CAD build for the part. Positions are in the model's coordinates, mm. Give positions to 0.01 mm unless a question says otherwise; leave off trailing zeros. Loops run counter-clockwise (first coordinate to the right, second up) from the corner with the lowest first, then second, coordinate; pieces in that order, holes last. Notation, with made-up numbers: (44, 43) -> (86, 43) arc R25 cw to (86, 76) -> close; hole circle Ø2 at (50, 19). An arc over 180 degrees is marked (long way). Use one line per item in the form item = value.
```python
from build123d import *

# Parameters (mm, degrees)
SKETCH1_W           = 245
SKETCH1_H           = 65
BOSS_EXTRUDE1_DEPTH = 3
CUT_EXTRUDE1_DEPTH  = 10
SKETCH3_W           = 3
SKETCH3_H           = 12.5
CUT_EXTRUDE2_DEPTH  = 10
SKETCH5_W           = 12
SKETCH5_H           = 3
SKETCH5_W_2         = 13.071416553
BOSS_EXTRUDE2_DEPTH = 3


with BuildPart() as part:
    # Sketch1 → Boss-Extrude1 (new body)
    with BuildSketch(Plane(origin=(0, 0, 0), x_dir=(1, 0, 0), z_dir=(0, 1, 0))):
        Rectangle(SKETCH1_W, SKETCH1_H)
    extrude(amount=BOSS_EXTRUDE1_DEPTH)

    # Sketch2 → Cut-Extrude1 (cut)
    with BuildSketch(Plane(origin=(0, 3, 0), x_dir=(1, 0, 0), z_dir=(0, 1, 0))):
        with BuildLine():
            Line((-85.5, 11), (-85.5, -11))
            ThreePointArc((-85.5, -11), (-96.5, -22), (-107.5, -11))
            Line((-107.5, -11), (-107.5, 11))
            ThreePointArc((-107.5, 11), (-96.5, 22), (-85.5, 11))
        make_face()
        with BuildLine():
            Line((86.035837844, -20), (76.144700887, -20))
            ThreePointArc((76.144700887, -20), (56.144700887, 0), (76.144700887, 20))
            Line((76.144700887, 20), (86.035837844, 20))
            ThreePointArc((86.035837844, 20), (106.035837844, 0), (86.035837844, -20))
        make_face()
        with BuildLine():
            Line((-64.530127929, 11), (-64.530127929, -11))
            ThreePointArc((-64.530127929, -11), (-53.530127929, -22), (-42.530127929, -11))
            Line((-42.530127929, -11), (-42.530127929, 11))
            ThreePointArc((-42.530127929, 11), (-53.530127929, 22), (-64.530127929, 11))
        make_face()
        with BuildLine():
            Line((-21.560255858, 11), (-21.560255858, -11))
            ThreePointArc((-21.560255858, -11), (-10.560255858, -22), (0.439744142, -11))
            Line((0.439744142, -11), (0.439744142, 11))
            ThreePointArc((0.439744142, 11), (-10.560255858, 22), (-21.560255858, 11))
        make_face()
        with BuildLine():
            Line((21.409616214, 11), (21.409616214, -11))
            ThreePointArc((21.409616214, -11), (32.409616214, -22), (43.409616214, -11))
            Line((43.409616214, -11), (43.409616214, 11))
            ThreePointArc((43.409616214, 11), (32.409616214, 22), (21.409616214, 11))
        make_face()
    extrude(amount=-CUT_EXTRUDE1_DEPTH, mode=Mode.SUBTRACT)

    # Sketch3 → Cut-Extrude2 (cut)
    with BuildSketch(Plane(origin=(0, 3, 0), x_dir=(1, 0, 0), z_dir=(0, 1, 0))):
        with Locations((121, 26.25)):
            Rectangle(SKETCH3_W, SKETCH3_H)
        with Locations((121, -26.25)):
            Rectangle(SKETCH3_W, SKETCH3_H)
    extrude(amount=-CUT_EXTRUDE2_DEPTH, mode=Mode.SUBTRACT)

    # Sketch5 → Boss-Extrude2 (add)
    with BuildSketch(Plane(origin=(0, 3, 0), x_dir=(1, 0, 0), z_dir=(0, 1, 0))):
        with Locations((58.5, 34)):
            Rectangle(SKETCH5_W, SKETCH5_H)
        with Locations((59.035708277, -34)):
            Rectangle(SKETCH5_W_2, SKETCH5_H)
    extrude(amount=-BOSS_EXTRUDE2_DEPTH)


solid = part.part
```
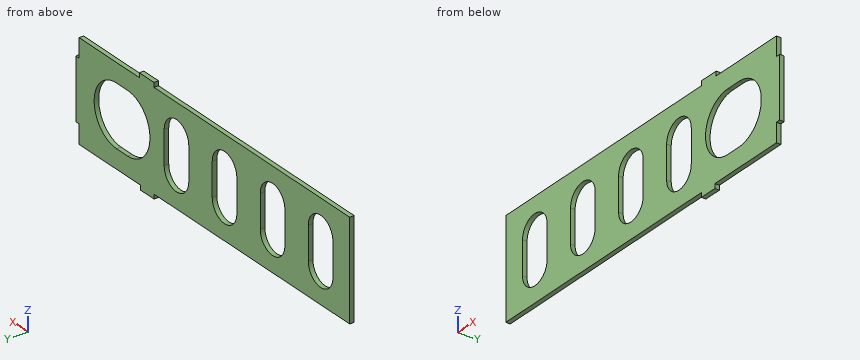
1. Drill centre lines: line 1 (X direction, y = 0.55, z = 13); line 2 (X direction, y = 1.65, z = 11.5); line 3 (X direction, y = 1.85, z = 27). Where is each one in solid material? Low to high.
Result sheet:
line_1 = -122.5 to -107.32, -85.68 to -64.35, -42.71 to -21.38, 0.26 to 21.59, 43.23 to 60.95, 101.23 to 122.5
line_2 = -122.5 to -107.49, -85.51 to -64.52, -42.54 to -21.55, 0.43 to 21.42, 43.4 to 59.78, 102.4 to 122.5
line_3 = -122.5 to 119.5
2. Cut at D-D, the plane y = 0.5. State how many separate pieces and enclosed holes the cut face has, then the cut area to 3 significant figures.
Result sheet:
separate_pieces = 1
enclosed_holes = 5
area = 10,800 mm^2
3. Drop flat-ended pins along their axis: P1, Ø4, axis at x = 17, z = 19.5, coming from the -Y side; P2, Ø0.9, axis at y = 2, z = -25, coming from the +X side; P3, Ø1.5, axis at x = 79.5, y = 1, coming from the +Z side; P4, Ø0.9, axis at x = -31, y = 1.5, coming from the -Z side. Give the stop position or say it passes through.
Result sheet:
P1 = 0
P2 = 119.5
P3 = 32.5
P4 = -32.5
4. Cut at C-C, the plane x = -18. Write the cut outline in (y, z).
Result sheet:
outline = (0, -32.5) -> (3, -32.5) -> (3, -19.1) -> (0, -19.1) -> close; (0, 19.1) -> (3, 19.1) -> (3, 32.5) -> (0, 32.5) -> close
5. Cut at A-A, the plane z = 0. Write the cut outline in (x, y), then the cut area to 3 significant figures.
Result sheet:
outline = (-122.5, 0) -> (-107.5, 0) -> (-107.5, 3) -> (-122.5, 3) -> close; (-85.5, 0) -> (-64.53, 0) -> (-64.53, 3) -> (-85.5, 3) -> close; (-42.53, 0) -> (-21.56, 0) -> (-21.56, 3) -> (-42.53, 3) -> close; (0.44, 0) -> (21.41, 0) -> (21.41, 3) -> (0.44, 3) -> close; (43.41, 0) -> (56.14, 0) -> (56.14, 3) -> (43.41, 3) -> close; (106.04, 0) -> (122.5, 0) -> (122.5, 3) -> (106.04, 3) -> close
area = 321 mm^2
6. Cut at B-B, the plane x = -96.5. Write the cut outline in (y, z), then the cut area to 3 significant figures.
Result sheet:
outline = (0, -32.5) -> (3, -32.5) -> (3, -22) -> (0, -22) -> close; (0, 22) -> (3, 22) -> (3, 32.5) -> (0, 32.5) -> close
area = 63.0 mm^2
